Source: CAD feature listing. Evaluate the final solid. Frame: model axes, mm. A direction names the side the tool comes from. Coordinates: 2 decimals unless noted, no trailing zeros. Loops run counter-clockwise (first coordinate to the right, second up) from the corner with the lowest first, then second, coordinate; pieces in that order, holes last. Notation, with made-up numbers: (44, -21) -> (74, -21) arc R25 cw to (74, -9) -> close; hole circle Ø1 at (38, 19). An arc over 180 degrees is marked (long way). One line per question, with ' | ' between items. Start each with the question number.
```python
from build123d import *

# Parameters (mm, degrees)
SKETCH1_W           = 19.05
SKETCH1_H           = 76.2
SKETCH1_W_2         = 13.05
SKETCH1_H_2         = 6.35
BOSS_EXTRUDE1_DEPTH = 10
SKETCH2_W           = 6.35
SKETCH2_H           = 35.4
BOSS_EXTRUDE2_DEPTH = 6.35
SKETCH3_R           = 2.25
CUT_EXTRUDE1_DEPTH  = 30


with BuildPart() as part:
    # Sketch1 → Boss-Extrude1 (new body)
    with BuildSketch(Plane.XY):
        with Locations((9.525, 38.1)):
            Rectangle(SKETCH1_W, SKETCH1_H)
        with Locations((9.525, 66.675)):
            Rectangle(SKETCH1_W_2, SKETCH1_H_2, mode=Mode.SUBTRACT)
        with Locations((9.525, 57.15)):
            Rectangle(SKETCH1_W_2, SKETCH1_H_2, mode=Mode.SUBTRACT)
        with Locations((9.525, 47.625)):
            Rectangle(SKETCH1_W_2, SKETCH1_H_2, mode=Mode.SUBTRACT)
        with Locations((9.525, 38.1)):
            Rectangle(SKETCH1_W_2, SKETCH1_H_2, mode=Mode.SUBTRACT)
        with Locations((9.525, 28.575)):
            Rectangle(SKETCH1_W_2, SKETCH1_H_2, mode=Mode.SUBTRACT)
        with Locations((9.525, 19.05)):
            Rectangle(SKETCH1_W_2, SKETCH1_H_2, mode=Mode.SUBTRACT)
        with Locations((9.525, 9.525)):
            Rectangle(SKETCH1_W_2, SKETCH1_H_2, mode=Mode.SUBTRACT)
    extrude(amount=BOSS_EXTRUDE1_DEPTH)

    # Sketch2 → Boss-Extrude2 (add)
    with BuildSketch(Plane.XZ):
        with Locations((3.175, 5)):
            Rectangle(SKETCH2_W, SKETCH2_H)
        with Locations((15.875, 5)):
            Rectangle(SKETCH2_W, SKETCH2_H)
    extrude(amount=BOSS_EXTRUDE2_DEPTH)

    # Sketch3 → Cut-Extrude1 (cut)
    with BuildSketch(Plane(origin=(19.05, 0, 0), x_dir=(0, 0, -1), z_dir=(1, 0, 0))):
        with Locations((-5, 66.675)):
            Circle(SKETCH3_R)
        with Locations((-5, 57.15)):
            Circle(SKETCH3_R)
        with Locations((-5, 47.625)):
            Circle(SKETCH3_R)
        with Locations((-5, 38.1)):
            Circle(SKETCH3_R)
        with Locations((-5, 28.575)):
            Circle(SKETCH3_R)
        with Locations((-5, 19.05)):
            Circle(SKETCH3_R)
        with Locations((-5, 9.525)):
            Circle(SKETCH3_R)
    extrude(amount=-CUT_EXTRUDE1_DEPTH, mode=Mode.SUBTRACT)


solid = part.part
```
(1) Cut plane D-D, the plane z = 5. State how many separate pieces and enclosed holes the cut face has, and give its area (3 significant figures).
(2) Access query for faces 1 (the flat face through (9, 41.275, 5)), 2 (the cylindrical face through (17.57, 26.58, 3.96)), 3 (the flat face through (3, 0, 16)). Directions: +Z, -Z, +X, -X, +Y, -Y. A direction counts if a zero-diameter tool reaches every point of the face in a straight line with its end or side. Return the directions, or none.
(3) Contact query for flat-ended pins moving along their axis: pin 1 Ø3 at (y, z) = (-4, -1.5) entering from -X; pin 2 Ø9.5 at (x, y) = (11, 51.5) entering from -Z; pin 3 Ø1.9 at (x, z) = (3, 17) entering from +Y; pin 4 Ø1.5 at (x, z) = (9.5, 11) entering from +Y. Output: stop coordinate, or through.
(4) Draft query along X for faces 4 (the cylindrical face through (1.52, 40.33, 5.29)), 5 (the flat face through (16.05, 27.8, 2.7)). Return one class per face: pulls with the +X half, pulls with the -X half, needs draft (parallel to the pull), parting line crosses it, or undercut.
(5) Cut plane A-A, the plane z = -1. Return the cut outline in (x, y).
(6) Ray query, L1, parallel to X at y = -2, z = 16; L2, parallel to X at y = 44.5, z = 9; L3, parallel to Y at x = 5.75, z = -4. Return the intervals inside material, ascending.
(7) Cut plane B-B, the plane y = 57.15. Return the cut outline in (x, z), and give its area (3 significant figures).
(8) Cut plane C-C, the plane x = 2. Return the cut outline in (y, z) (3 decimals), and give its area (3 significant figures).
Here are the results:
1) separate pieces: 8 | enclosed holes: 0 | area: 763 mm2
2) face 1: +Z, -Z | face 2: +X, -X | face 3: +Z, +X, -X, +Y
3) pin 1: stops at x = 0 | pin 2: stops at z = 0 | pin 3: stops at y = 0 | pin 4: passes through
4) face 4: needs draft | face 5: undercut
5) outline: (0, -6.35) -> (6.35, -6.35) -> (6.35, 0) -> (0, 0) -> close; (12.7, -6.35) -> (19.05, -6.35) -> (19.05, 0) -> (12.7, 0) -> close
6) L1: x = 0 to 6.35, 12.7 to 19.05 | L2: x = 0 to 3, 16.05 to 19.05 | L3: y = -6.35 to 0
7) outline: (0, 0) -> (3, 0) -> (3, 2.75) -> (0, 2.75) -> close; (0, 7.25) -> (3, 7.25) -> (3, 10) -> (0, 10) -> close; (16.05, 0) -> (19.05, 0) -> (19.05, 2.75) -> (16.05, 2.75) -> close; (16.05, 7.25) -> (19.05, 7.25) -> (19.05, 10) -> (16.05, 10) -> close | area: 33.0 mm2
8) outline: (-6.35, -12.7) -> (0, -12.7) -> (0, 0) -> (76.2, 0) -> (76.2, 10) -> (0, 10) -> (0, 22.7) -> (-6.35, 22.7) -> close; hole circle Ø4.5 at (9.525, 5); hole circle Ø4.5 at (19.05, 5); hole circle Ø4.5 at (28.575, 5); hole circle Ø4.5 at (38.1, 5); hole circle Ø4.5 at (47.625, 5); hole circle Ø4.5 at (57.15, 5); hole circle Ø4.5 at (66.675, 5) | area: 875 mm2
